from build123d import *

# Parameters (mm, degrees)
F0_W     = 152.4
F0_H     = 76.2
F1_DEPTH = 25.4
F2_R     = 5.08
F3_T     = -2.032


with BuildPart() as f1:
    # F0 (on Top) → F1 (new body)
    with BuildSketch(Plane.XY):
        with Locations((-82.550001, 38.1)):
            Rectangle(F0_W, F0_H)
    extrude(amount=F1_DEPTH)

    # F2
    f2_edges = [f1.edges().sort_by_distance(p)[0] for p in [
        (-158.750001, 0, 12.7),
        (-6.350001, 0, 12.7),
        (-158.750001, 76.2, 12.7),
        (-6.350001, 76.2, 12.7),
    ]]
    fillet(f2_edges, radius=F2_R)

    # F3
    f3_openings = [f1.faces().sort_by_distance(p)[0] for p in [
        (-82.550001, 38.1, 25.4),
    ]]
    offset(amount=F3_T, openings=f3_openings)


solid = f1.part
Read the model definition and answer for the solid it produces. Units are mm, in the model's axes. A direction names the side the tool comes from. Coordinates: 2 decimals unless noted, no trailing zeros. Loops run counter-clockwise (first coordinate to the right, second up) from the corner with the lowest first, then second, coordinate; pieces in that order, holes last.
Q1. The part is cut by section A-A on z = 20.5. Write down the section's boundary in (x, y).
Q2. Which of the six approach directions +Z, -Z, +X, -X, +Y, -Y give full straight-line access (tool end or side, diameter ignored) to faces 1 (the face through (-9.3, 73.3, 13.9)), 2 (the face through (-7.878, 1.449, 12.878))?
Q3. This flat-tipped pin is pushed along its axis until it touches: pin 1 Ø12 at (x, y) = (-44, 14) entering from +Z. Where does it stop, or does it pass through?
Q4. The mould has two halves that part along X. Classify faces 3 (the face through (-156.718, 38, 14)), 4 (the face through (-157.301, 1.528, 12.878)), 5 (the face through (-84, 39, 0)): +X half, -X half, draft (parallel to the pull), parting line (faces both ways), or undercut.
Q5. The part is cut by section C-C on y = 40. Write down the section's boundary in (x, z), and give its area (3 significant figures).
Q6. The part is cut by section B-B on x = -89. Write down the section's boundary in (y, z), and give its area (3 significant figures).
Q7. Consider probe 1 along X at (y, z) = (63, 4); probe 2 along Y at (x, z) = (-129.5, 17); probe 3 along Z at (x, y) = (-85, 67). Determine where each line is inside the solid, lowest interval first.
Results below:
1. outline: (-158.75, 5.08) arc R5.08 ccw to (-153.67, 0) - (-11.43, 0) arc R5.08 ccw to (-6.35, 5.08) - (-6.35, 71.12) arc R5.08 ccw to (-11.43, 76.2) - (-153.67, 76.2) arc R5.08 ccw to (-158.75, 71.12) - close; hole (-156.72, 5.08) arc R3.05 ccw to (-153.67, 2.03) - (-11.43, 2.03) arc R3.05 ccw to (-8.38, 5.08) - (-8.38, 71.12) arc R3.05 ccw to (-11.43, 74.17) - (-153.67, 74.17) arc R3.05 ccw to (-156.72, 71.12) - close
2. face 1: +Z
2. face 2: +Z, -Z, +X, -Y
3. pin 1: stops at z = 2.03
4. face 3: undercut
4. face 4: -X half
4. face 5: draft
5. outline: (-158.75, 0) - (-6.35, 0) - (-6.35, 25.4) - (-8.38, 25.4) - (-8.38, 2.03) - (-156.72, 2.03) - (-156.72, 25.4) - (-158.75, 25.4) - close
5. area: 405 mm2
6. outline: (0, 0) - (76.2, 0) - (76.2, 25.4) - (74.17, 25.4) - (74.17, 2.03) - (2.03, 2.03) - (2.03, 25.4) - (0, 25.4) - close
6. area: 250 mm2
7. probe 1: x = -158.75 to -156.72, -8.38 to -6.35
7. probe 2: y = 0 to 2.03, 74.17 to 76.2
7. probe 3: z = 0 to 2.03
